Can you work these out from the model? Positions are in its coordinate system, mm. A direction names the side the tool comes from. Round coordinates to 2 decimals unless told otherwise and drop trailing zeros. Order: outer loops, then holes, each group sorted by start corner. A loop starts at its lowest first (then second) coordinate and runs counter-clockwise, first axis right, second up. Notation, with made-up numbers: (49.5, 20.25) -> (53.5, 20.25) arc R14 cw to (53.5, 24.25) -> close; hole circle Ø9 at (-34, 73). An arc over 180 degrees is marked (long way). Use a Markdown table: item, result. Add a question column.
Q1. If we section it at A-A on x = -13: List the corners of the cut face in (y, z) for me.
Q2. For faces 1 (the face through (41.5, -0.4, -0.1)), 2 (the face through (-1, 0, 13)), 3 (the face through (1, 2, -4.732)), which set-ups out of +Z, -Z, +X, -X, +Y, -Y let a thin tool reach every point of the face, with its end or its side?
Q3. I'm going to push a flat-ended pin straight in: pin 1 Ø11.5 at (x, z) = (-8, -15) entering from +Y. Where does the tip first touch, or does it pass through?
Q4. If we section it at C-C on y = 1.5: List the corners of the cut face in (x, z) for me, plus the area to 3 significant figures.
Q5. If we section it at B-B on z = 21: List the corners of the cut face in (x, y) for me.
Q6. I need wall thicknesses on line 1 along Y through (x, z) = (33, 20); line 2 along Z through (x, y) = (4, 1.1). Which ranges of each line are inside material? Lowest first, please. Write a range as [from, to].
```python
from build123d import *

# Parameters (mm, degrees)
F0_W     = 83
F0_H     = 56
F1_DEPTH = 1
F3_DEPTH = 83


# Not quite as in the source:
# - a feature names something its author has since deleted; it is built from what else it names


with BuildPart() as f1:
    # F0 (on Front) → F1 (new body)
    with BuildSketch(Plane.XZ):
        Rectangle(F0_W, F0_H)
    extrude(amount=F1_DEPTH)

    # F2 (on face) → F3 (join)
    with BuildSketch(Plane.YZ.offset(41.5)):
        with BuildLine():
            ThreePointArc((3.3219824545, -3.733111607), (3.130625787, -3), (3.3219824545, -2.266888393))
            Line((3.3219824545, -2.266888393), (3.3219824545, -1.492598909))
            Line((3.3219824545, -1.492598909), (0, -1.492598909))
            Line((0, -1.492598909), (0, -4.7320667654))
            Line((0, -4.7320667654), (3.3219824545, -4.7320667654))
            Line((3.3219824545, -4.7320667654), (3.3219824545, -3.733111607))
        make_face()
        with BuildLine():
            ThreePointArc((0, 27.0385164807), (-0.1, 26.5), (0, 25.9614835193))
            Line((0, 25.9614835193), (0, 27.0385164807))
        make_face()
    extrude(amount=-F3_DEPTH)


solid = f1.part
```
Answer below:
| question | item | result |
|---|---|---|
| 1 | outline | (-1, -28) -> (0, -28) -> (0, -4.73) -> (3.32, -4.73) -> (3.32, -3.73) arc R1.5 cw to (3.32, -2.27) -> (3.32, -1.49) -> (0, -1.49) -> (0, 28) -> (-1, 28) -> close |
| 2 | face 1 | +Z, -Z, +X, +Y, -Y |
| 2 | face 2 | +Z, +X, -X, +Y |
| 2 | face 3 | -Z, +X, -X, +Y |
| 3 | pin 1 | y = 0 |
| 4 | outline | (-41.5, -4.73) -> (41.5, -4.73) -> (41.5, -1.49) -> (-41.5, -1.49) -> close |
| 4 | area | 269 mm² |
| 5 | outline | (-41.5, -1) -> (41.5, -1) -> (41.5, 0) -> (-41.5, 0) -> close |
| 6 | line 1 | [-1, 0] |
| 6 | line 2 | [-4.73, -1.49] |
